Could you check a few things on this model? Use its own coordinates, in mm. A direction names the side the tool comes from. Give positions to 0.01 mm unless a question says otherwise; leave off trailing zeros. Order: outer loops, then holes, each group sorted by start corner. A loop starts at its lowest first (then second) coordinate and runs counter-clockwise, first axis right, second up. Notation, with made-up numbers: M 46,-37 L 95,-37 A12 ccw 95,-19 Z; hole C 50.25,87.25 d10. An arc over 180 degrees is marked long. Return JSON: item names as keys, results as strings. Group by question number.
```python
from build123d import *

# Parameters (mm, degrees)
SKETCH1_W           = 3.81
SKETCH1_H           = 12.7
SKETCH2_R           = 1.778
CUT_EXTRUDE1_DEPTH  = 15.24
SKETCH3_R           = 1.778
CUT_EXTRUDE2_DEPTH  = 4.81
SKETCH6_W           = 7.62
SKETCH6_H           = 3.81
BOSS_EXTRUDE1_DEPTH = 10.922
CUT_EXTRUDE3_DEPTH  = 6.096


with BuildPart() as part:
    # Sketch1 → Revolve1 (revolve)
    with BuildSketch(Plane(origin=(0, 0, 0), x_dir=(0, 0, -1), z_dir=(1, 0, 0)), mode=Mode.PRIVATE) as revolve1_sk:
        with Locations((-1.905, 136.398)):
            Rectangle(SKETCH1_W, SKETCH1_H)
    revolve(revolve1_sk.sketch.rotate(Axis((0, 0, 0), (0, 0, -1)), 90), axis=Axis((0, 0, 0), (0, 0, -1)))  # turned: the seam where the file's is

    # Sketch2 → Cut-Extrude1 (cut, symmetric)
    with BuildSketch(Plane.XY.offset(3.81)):
        with Locations((0, 137.668)):
            Circle(SKETCH2_R)
        with Locations((107.633176528, 85.834594042)):
            Circle(SKETCH2_R)
        with Locations((134.216375814, -30.634011936)):
            Circle(SKETCH2_R)
        with Locations((59.731906597, -124.034582106)):
            Circle(SKETCH2_R)
        with Locations((-59.731906597, -124.034582106)):
            Circle(SKETCH2_R)
        with Locations((-134.216375814, -30.634011936)):
            Circle(SKETCH2_R)
        with Locations((-107.633176528, 85.834594042)):
            Circle(SKETCH2_R)
    extrude(amount=CUT_EXTRUDE1_DEPTH, both=True, mode=Mode.SUBTRACT)

    # Sketch3 → Cut-Extrude2 (cut, through all)
    with BuildSketch(Plane.XY.offset(3.81)):
        with BuildLine():
            ThreePointArc((-70.003567413, -116.471424175), (-72.443427116, -117.079414825), (-71.835436467, -119.519274528))
            ThreePointArc((-71.835436467, -119.519274528), (-66.24004713, -122.708773411), (-60.503351759, -125.636504814))
            ThreePointArc((-60.503351759, -125.636504814), (-61.333829237, -123.263136804), (-58.960461155, -122.432659533))
            ThreePointArc((-58.960461155, -122.432659533), (-64.550865586, -119.579587941), (-70.003567413, -116.471424175))
        make_face()
        with BuildLine():
            ThreePointArc((-57.953906597, -124.034582106), (-58.785953505, -125.540057695), (-60.503351759, -125.636504814))
            ThreePointArc((-60.503351759, -125.636504814), (-54.637588239, -128.296223122), (-48.655269538, -130.68225458))
            ThreePointArc((-48.655269538, -130.68225458), (-46.36863444, -129.636373168), (-47.414515852, -127.34973807))
            ThreePointArc((-47.414515852, -127.34973807), (-53.244279962, -125.024552594), (-58.960461155, -122.432659533))
            ThreePointArc((-58.960461155, -122.432659533), (-58.226430925, -123.088629147), (-57.953906597, -124.034582106))
        make_face()
        with BuildLine():
            ThreePointArc((47.414515852, -127.34973807), (46.36863444, -129.636373168), (48.655269538, -130.68225458))
            ThreePointArc((48.655269538, -130.68225458), (54.637588297, -128.296223097), (60.503351873, -125.636504759))
            ThreePointArc((60.503351873, -125.636504759), (58.129983953, -124.806027402), (58.960461282, -122.432659472))
            ThreePointArc((58.960461282, -122.432659472), (53.244280027, -125.024552566), (47.414515852, -127.34973807))
        make_face()
        with BuildLine():
            ThreePointArc((61.509906597, -124.034582106), (61.23738222, -124.980535144), (60.503351873, -125.636504759))
            ThreePointArc((60.503351873, -125.636504759), (66.240047187, -122.708773381), (71.835436467, -119.519274528))
            ThreePointArc((71.835436467, -119.519274528), (72.443427116, -117.079414825), (70.003567413, -116.471424175))
            ThreePointArc((70.003567413, -116.471424175), (64.550865648, -119.579587907), (58.960461282, -122.432659472))
            ThreePointArc((58.960461282, -122.432659472), (60.677859616, -122.529106472), (61.509906597, -124.034582106))
        make_face()
        with BuildLine():
            ThreePointArc((-72.088346147, -123.208205302), (-74.362361234, -114.520636287), (-65.67479222, -112.2466212))
            ThreePointArc((-65.67479222, -112.2466212), (-64.697785609, 112.812582815), (130.048, 0))
            ThreePointArc((130.048, 0), (112.812582815, -64.697785609), (65.67479222, -112.2466212))
            ThreePointArc((65.67479222, -112.2466212), (74.362361234, -114.520636287), (72.088346147, -123.208205302))
            ThreePointArc((72.088346147, -123.208205302), (123.829436605, -71.015928735), (142.748, 0))
            ThreePointArc((142.748, 0), (-71.015928735, 123.829436605), (-72.088346147, -123.208205302))
        make_face()
        with Locations((-134.216375814, -30.634011936)):
            Circle(SKETCH3_R, mode=Mode.SUBTRACT)
        with Locations((134.216375814, -30.634011936)):
            Circle(SKETCH3_R, mode=Mode.SUBTRACT)
        with Locations((-107.633176528, 85.834594042)):
            Circle(SKETCH3_R, mode=Mode.SUBTRACT)
        with Locations((0, 137.668)):
            Circle(SKETCH3_R, mode=Mode.SUBTRACT)
        with Locations((107.633176528, 85.834594042)):
            Circle(SKETCH3_R, mode=Mode.SUBTRACT)
    extrude(amount=-CUT_EXTRUDE2_DEPTH, mode=Mode.SUBTRACT)

    # Sketch6 → Boss-Extrude1 (add)
    with BuildSketch(Plane.XZ.offset(130.048)):
        with Locations((0, 1.905)):
            Rectangle(SKETCH6_W, SKETCH6_H)
    extrude(amount=-BOSS_EXTRUDE1_DEPTH)

    # Sketch7 → Cut-Extrude3 (cut)
    with BuildSketch(Plane(origin=(0, -119.126, 0), x_dir=(1, 0, 0), z_dir=(0, 1, 0))):
        Polygon((-1.27, 0), (-2.032, -0.635), (-2.032, -1.651), (2.032, -1.651), (2.032, -0.635), (1.27, 0), align=None)
    extrude(amount=-CUT_EXTRUDE3_DEPTH, mode=Mode.SUBTRACT)


solid = part.part
```
1. For pin 1 (1 mm diameter, centred on x = 21, z = 2.5, fed in from +Y); pin 2 (1.1 mm diameter, centred on y = -123.5, z = 1.5, fed in from +X); pin 3 (1.9 mm diameter, centred on y = -123.5, z = 1, fed in from +X); pin 4 (3.5 mm diameter, centred on x = 0, y = -122, fed in from -Z), each with a flat end and sliding along its axis, tell me the tip position at first contact or that it passes through.
2. Imagine slicing it at A-A, the plane x = -57.5. Please give me the cut outline in (y, z).
3. Imagine slicing it at C-C, the plane x = 5.5. Please give me the cut outline in (y, z), plus the area to 3 significant figures.
4. Which directions (+Z, -Z, +X, -X, +Y, -Y) give clear straight access to the entire face, cutting with the end or side of a thin tool? Please do faces 5 (the flat face through (0, -119.126, 2)), 6 (the cylindrical face through (72.46, -117.11, 1.93)).
5. Imagine slicing it at B-B, the plane y = -133. Please give me the cut outline in (x, z), plus the area to 3 significant figures.
6. If we mould it in two halves opening along Z, with no side actions, what happens to faces 1 (the flat face through (0, -122, 1.651)), 2 (the flat face through (-1, -131, 0)), 3 (the cylindrical face through (-46.38, -129.67, 1.93)), 4 (the flat face through (1, -131, 3.81))? For each: pulls with the +Z half, pulls with the -Z half, needs draft (parallel to the pull), parting line crosses it, or undercut.
7. I need wall thicknesses on L1, parallel to X at y = -117.5, z = 3.4; L2, parallel to X at y = -116.5, z = 1.2; L3, parallel to Y at x = -2.5, z = 2.75. Which ranges of each line are inside material? Lowest first, please. Write a range as from..to.
Values:
{
 "1": {"pin 1": "stops at y = -128.26", "pin 2": "stops at x = 72.49", "pin 3": "stops at x = 73.01", "pin 4": "stops at z = 0"},
 "2": {"outline": "M -130.66,0 L -127.04,0 L -127.04,3.81 L -130.66,3.81 Z; M -123.13,0 L -116.65,0 L -116.65,3.81 L -123.13,3.81 Z"},
 "3": {"outline": "M -142.64,0 L -129.93,0 L -129.93,3.81 L -142.64,3.81 Z", "area": "48.4 mm²"},
 "4": {"face 5": "+Z, -Z, +Y", "face 6": "+Z, -Z"},
 "5": {"outline": "M -51.85,0 L 51.85,0 L 51.85,3.81 L -51.85,3.81 Z", "area": "395 mm²"},
 "6": {"face 1": "undercut", "face 2": "pulls with the -Z half", "face 3": "needs draft", "face 4": "pulls with the +Z half"},
 "7": {"L1": "x = -75.23..-72.63, -68.26..-55.73, 55.73..68.26, 72.63..75.23", "L2": "x = -75.11..-71.88, -69.96..-57.79, 57.79..69.96, 71.88..75.11", "L3": "y = -142.73..-119.13"}
}
